For this review, take the finished solid that the model builds, in its own axes (mm). Give positions to 0.01 mm unless a question says otherwise; leave off trailing zeros. Order: outer loops, then holes, each group sorted by start corner. A loop starts at its lowest first (then second) coordinate and runs counter-clockwise, first axis right, second up.
from build123d import *

# Parameters (mm, degrees)
SKETCH1_W                = 210
SKETCH1_H                = 70
BOSS_EXTRUDE1_DEPTH      = 3
SKETCH2_W                = 10
SKETCH2_H                = 3
CUT_EXTRUDE1_DEPTH       = 3
LPATTERN1_COUNT          = 11
LPATTERN1_PITCH          = 20
MIRROR1_COPY_1_SKETCH_W  = 10
MIRROR1_COPY_1_SKETCH_H  = 3
MIRROR1_COPY_1_DEPTH     = 3
MIRROR1_COPY_2_SKETCH_W  = 10
MIRROR1_COPY_2_SKETCH_H  = 3
MIRROR1_COPY_2_DEPTH     = 3
MIRROR1_COPY_3_SKETCH_W  = 10
MIRROR1_COPY_3_SKETCH_H  = 3
MIRROR1_COPY_3_DEPTH     = 3
MIRROR1_COPY_4_SKETCH_W  = 10
MIRROR1_COPY_4_SKETCH_H  = 3
MIRROR1_COPY_4_DEPTH     = 3
MIRROR1_COPY_5_SKETCH_W  = 10
MIRROR1_COPY_5_SKETCH_H  = 3
MIRROR1_COPY_5_DEPTH     = 3
MIRROR1_COPY_6_SKETCH_W  = 10
MIRROR1_COPY_6_SKETCH_H  = 3
MIRROR1_COPY_6_DEPTH     = 3
MIRROR1_COPY_7_SKETCH_W  = 10
MIRROR1_COPY_7_SKETCH_H  = 3
MIRROR1_COPY_7_DEPTH     = 3
MIRROR1_COPY_8_SKETCH_W  = 10
MIRROR1_COPY_8_SKETCH_H  = 3
MIRROR1_COPY_8_DEPTH     = 3
MIRROR1_COPY_9_SKETCH_W  = 10
MIRROR1_COPY_9_SKETCH_H  = 3
MIRROR1_COPY_9_DEPTH     = 3
MIRROR1_COPY_10_SKETCH_W = 10
MIRROR1_COPY_10_SKETCH_H = 3
MIRROR1_COPY_10_DEPTH    = 3
SKETCH3_W                = 3
SKETCH3_H                = 10
CUT_EXTRUDE2_DEPTH       = 3
LPATTERN2_COUNT          = 3
LPATTERN2_PITCH          = 20
MIRROR2_COPY_1_SKETCH_W  = 3
MIRROR2_COPY_1_SKETCH_H  = 10
MIRROR2_COPY_1_DEPTH     = 3
MIRROR2_COPY_2_SKETCH_W  = 3
MIRROR2_COPY_2_SKETCH_H  = 10
MIRROR2_COPY_2_DEPTH     = 3


with BuildPart() as part:
    # Sketch1 → Boss-Extrude1 (new body)
    with BuildSketch(Plane(origin=(0, 0, 0), x_dir=(0, 0, -1), z_dir=(1, 0, 0))):
        Rectangle(SKETCH1_W, SKETCH1_H)
    extrude(amount=BOSS_EXTRUDE1_DEPTH)

    # Sketch2 → Cut-Extrude1 (cut)
    with BuildSketch(Plane(origin=(3, 0, 0), x_dir=(0, 0, -1), z_dir=(1, 0, 0))):
        with Locations((-100, 33.5)):
            Rectangle(SKETCH2_W, SKETCH2_H)
    cut_extrude1 = extrude(amount=-CUT_EXTRUDE1_DEPTH, mode=Mode.SUBTRACT)

    # LPattern1: Cut-Extrude1 ×11
    with Locations(*[(0, 0, -i * LPATTERN1_PITCH) for i in range(1, LPATTERN1_COUNT)]):
        add(cut_extrude1, mode=Mode.SUBTRACT)

    # Mirror1: Cut-Extrude1 across plane
    add(cut_extrude1.mirror(Plane.ZX), mode=Mode.SUBTRACT)

    # Mirror1 copy 1 sketch → Mirror1 copy 1 (cut)
    with BuildSketch(Plane(origin=(3, 0, -20), x_dir=(0, 0, -1), z_dir=(1, 0, 0))):
        with Locations((-100, -33.5)):
            Rectangle(MIRROR1_COPY_1_SKETCH_W, MIRROR1_COPY_1_SKETCH_H)
    extrude(amount=-MIRROR1_COPY_1_DEPTH, mode=Mode.SUBTRACT)

    # Mirror1 copy 2 sketch → Mirror1 copy 2 (cut)
    with BuildSketch(Plane(origin=(3, 0, -40), x_dir=(0, 0, -1), z_dir=(1, 0, 0))):
        with Locations((-100, -33.5)):
            Rectangle(MIRROR1_COPY_2_SKETCH_W, MIRROR1_COPY_2_SKETCH_H)
    extrude(amount=-MIRROR1_COPY_2_DEPTH, mode=Mode.SUBTRACT)

    # Mirror1 copy 3 sketch → Mirror1 copy 3 (cut)
    with BuildSketch(Plane(origin=(3, 0, -60), x_dir=(0, 0, -1), z_dir=(1, 0, 0))):
        with Locations((-100, -33.5)):
            Rectangle(MIRROR1_COPY_3_SKETCH_W, MIRROR1_COPY_3_SKETCH_H)
    extrude(amount=-MIRROR1_COPY_3_DEPTH, mode=Mode.SUBTRACT)

    # Mirror1 copy 4 sketch → Mirror1 copy 4 (cut)
    with BuildSketch(Plane(origin=(3, 0, -80), x_dir=(0, 0, -1), z_dir=(1, 0, 0))):
        with Locations((-100, -33.5)):
            Rectangle(MIRROR1_COPY_4_SKETCH_W, MIRROR1_COPY_4_SKETCH_H)
    extrude(amount=-MIRROR1_COPY_4_DEPTH, mode=Mode.SUBTRACT)

    # Mirror1 copy 5 sketch → Mirror1 copy 5 (cut)
    with BuildSketch(Plane(origin=(3, 0, -100), x_dir=(0, 0, -1), z_dir=(1, 0, 0))):
        with Locations((-100, -33.5)):
            Rectangle(MIRROR1_COPY_5_SKETCH_W, MIRROR1_COPY_5_SKETCH_H)
    extrude(amount=-MIRROR1_COPY_5_DEPTH, mode=Mode.SUBTRACT)

    # Mirror1 copy 6 sketch → Mirror1 copy 6 (cut)
    with BuildSketch(Plane(origin=(3, 0, -120), x_dir=(0, 0, -1), z_dir=(1, 0, 0))):
        with Locations((-100, -33.5)):
            Rectangle(MIRROR1_COPY_6_SKETCH_W, MIRROR1_COPY_6_SKETCH_H)
    extrude(amount=-MIRROR1_COPY_6_DEPTH, mode=Mode.SUBTRACT)

    # Mirror1 copy 7 sketch → Mirror1 copy 7 (cut)
    with BuildSketch(Plane(origin=(3, 0, -140), x_dir=(0, 0, -1), z_dir=(1, 0, 0))):
        with Locations((-100, -33.5)):
            Rectangle(MIRROR1_COPY_7_SKETCH_W, MIRROR1_COPY_7_SKETCH_H)
    extrude(amount=-MIRROR1_COPY_7_DEPTH, mode=Mode.SUBTRACT)

    # Mirror1 copy 8 sketch → Mirror1 copy 8 (cut)
    with BuildSketch(Plane(origin=(3, 0, -160), x_dir=(0, 0, -1), z_dir=(1, 0, 0))):
        with Locations((-100, -33.5)):
            Rectangle(MIRROR1_COPY_8_SKETCH_W, MIRROR1_COPY_8_SKETCH_H)
    extrude(amount=-MIRROR1_COPY_8_DEPTH, mode=Mode.SUBTRACT)

    # Mirror1 copy 9 sketch → Mirror1 copy 9 (cut)
    with BuildSketch(Plane(origin=(3, 0, -180), x_dir=(0, 0, -1), z_dir=(1, 0, 0))):
        with Locations((-100, -33.5)):
            Rectangle(MIRROR1_COPY_9_SKETCH_W, MIRROR1_COPY_9_SKETCH_H)
    extrude(amount=-MIRROR1_COPY_9_DEPTH, mode=Mode.SUBTRACT)

    # Mirror1 copy 10 sketch → Mirror1 copy 10 (cut)
    with BuildSketch(Plane(origin=(3, 0, -200), x_dir=(0, 0, -1), z_dir=(1, 0, 0))):
        with Locations((-100, -33.5)):
            Rectangle(MIRROR1_COPY_10_SKETCH_W, MIRROR1_COPY_10_SKETCH_H)
    extrude(amount=-MIRROR1_COPY_10_DEPTH, mode=Mode.SUBTRACT)

    # Sketch3 → Cut-Extrude2 (cut)
    with BuildSketch(Plane(origin=(3, 0, 0), x_dir=(0, 0, -1), z_dir=(1, 0, 0))):
        with Locations((-103.5, 20)):
            Rectangle(SKETCH3_W, SKETCH3_H)
    cut_extrude2 = extrude(amount=-CUT_EXTRUDE2_DEPTH, mode=Mode.SUBTRACT)

    # LPattern2: Cut-Extrude2 ×3
    with Locations(*[(0, -i * LPATTERN2_PITCH, 0) for i in range(1, LPATTERN2_COUNT)]):
        add(cut_extrude2, mode=Mode.SUBTRACT)

    # Mirror2: Cut-Extrude2 across plane
    add(cut_extrude2.mirror(Plane.XY), mode=Mode.SUBTRACT)

    # Mirror2 copy 1 sketch → Mirror2 copy 1 (cut)
    with BuildSketch(Plane(origin=(3, -20, 0), x_dir=(0, 0, 1), z_dir=(1, 0, 0))):
        with Locations((-103.5, -20)):
            Rectangle(MIRROR2_COPY_1_SKETCH_W, MIRROR2_COPY_1_SKETCH_H)
    extrude(amount=-MIRROR2_COPY_1_DEPTH, mode=Mode.SUBTRACT)

    # Mirror2 copy 2 sketch → Mirror2 copy 2 (cut)
    with BuildSketch(Plane(origin=(3, -40, 0), x_dir=(0, 0, 1), z_dir=(1, 0, 0))):
        with Locations((-103.5, -20)):
            Rectangle(MIRROR2_COPY_2_SKETCH_W, MIRROR2_COPY_2_SKETCH_H)
    extrude(amount=-MIRROR2_COPY_2_DEPTH, mode=Mode.SUBTRACT)


solid = part.part
1) Clearance check with flat-ended pins moving along their axes: pin 1 (0.9 mm diameter, centred on x = 1.5, y = -33, fed in from +Z); pin 2 (1.5 mm diameter, centred on x = 1.5, y = 33, fed in from -Z); pin 3 (0.9 mm diameter, centred on x = 1, z = 103.5, fed in from +Y). State where each tip first meets the part, or that it passes through.
Answer sheet:
pin 1: stops at z = 95
pin 2: stops at z = -95
pin 3: stops at y = 32
2) We need section B-B on z = 58. Give the boundary of the cut face in (x, y).
Answer sheet:
outline: (0, -32) - (3, -32) - (3, 32) - (0, 32) - close
3) We need section A-A on y = 21. Give the boundary of the cut face in (x, z).
Answer sheet:
outline: (0, -102) - (3, -102) - (3, 102) - (0, 102) - close
4) To check wall thickness, follow line 1 (Z direction, x = 2.5, y = -1); line 2 (Y direction, x = 1.2, z = 24). State the ranges of each line that lie inside material, in increasing order.
Answer sheet:
line 1: z = -102 to 102
line 2: y = -32 to 32
